The listing builds one solid part. Answer for the finished solid, in the listing's coordinates (mm). A direction names the side the tool comes from. Give positions to 0.01 mm unless a question says otherwise; leave off trailing zeros. Order: outer loops, then holes, each group sorted by start corner. A loop starts at its lowest first (then second) coordinate and runs counter-clockwise, first axis right, second up.
```python
from build123d import *

# Parameters (mm, degrees)
M5X0_8_1_AT_2_COUNT = 2
M5X0_8_1_AT_2_PITCH = 90.280227073


with BuildPart() as part:
    # 草图2 → 旋转4 (revolve)
    with BuildSketch(Plane(origin=(0, 0, 0), x_dir=(0, 0, -1), z_dir=(1, 0, 0)), mode=Mode.PRIVATE) as revolve_4_sk:
        Polygon((27.5, 94), (26, 94), (26, 96), (-26, 96), (-26, 94), (-27.5, 94), (-27.5, 90), (27.5, 90), align=None)
    revolve(revolve_4_sk.sketch.rotate(Axis((0, 90, -27.5), (0, 0, 1)), 90), axis=Axis((0, 90, -27.5), (0, 0, 1)))

    # 草图5 → M5x0.8 螺纹孔的螺纹孔钻头1 (revolve, cut)
    with BuildSketch(Plane(origin=(0, 90, 27.5), x_dir=(0, -1, 0), z_dir=(1, 0, 0))):
        Polygon((0, 0), (0, 16.2618073), (2.1, 15), (2.1, 0), align=None)
    m5x0_8_1 = revolve(axis=Axis((0, 90, 33.85), (0, 0, -1)), mode=Mode.SUBTRACT)

    # M5x0.8 螺纹孔的螺纹孔钻头1 at 2: M5x0.8 螺纹孔的螺纹孔钻头1 ×2
    with Locations(*[Vector(-0.6431998246516509, -0.765698364611082, 0) * (i * M5X0_8_1_AT_2_PITCH) for i in range(1, M5X0_8_1_AT_2_COUNT)]):
        add(m5x0_8_1, mode=Mode.SUBTRACT)

    # 镜向1: M5x0.8 螺纹孔的螺纹孔钻头1 across plane
    add(m5x0_8_1.mirror(Plane.XY), mode=Mode.SUBTRACT)

    # 镜向1 copy 1 sketch → 镜向1 copy 1 (revolve, cut)
    with BuildSketch(Plane(origin=(-58.068226223, 20.872577773, -27.5), x_dir=(0, -1, 0), z_dir=(1, 0, 0))):
        Polygon((0, 0), (0, -16.2618073), (2.1, -15), (2.1, 0), align=None)
    revolve(axis=Axis((-58.068226223, 20.872577773, -33.85), (0, 0, -1)), mode=Mode.SUBTRACT)


solid = part.part
```
1) Given P1, Ø5.5, axis at x = 0, y = 90, coming from the -Z side; P2, Ø1, axis at x = 1.5, z = 6.5, coming from the +Y side; P3, Ø2, axis at y = 93.5, z = 9, coming from the -X side; P4, Ø3, axis at x = 2, z = -18, coming from the -Y side, each flat-ended and moving along its own axis, determine where each tip first touches the part or whether it passes through.
Geometry says:
P1: stops at z = -27.5
P2: stops at y = 95.92
P3: stops at x = -5.45
P4: stops at y = 84.02
2) Find section B-B (x = -3.25). Write down the section's boundary in (y, z), then the cut area to 3 significant figures.
Geometry says:
outline: (84.96, -26) - (87.67, -26) - (87.67, -27.5) - (92.33, -27.5) - (92.33, -26) - (95.04, -26) - (95.04, 26) - (92.33, 26) - (92.33, 27.5) - (87.67, 27.5) - (87.67, 26) - (84.96, 26) - close
area: 539 mm2
3) A tool of negligible diameter and unlimited length cuts with its end or side. For faces 4 (the cylindrical face through (-0.09, 92.1, 20.1)), 5 (the cylindrical face through (0.867, 93.905, -26.74)), 6 (the flat face through (2, 92, -27.5)), from which of +Z, -Z, +X, -X, +Y, -Y can it reach the whole face along a straight path? Write none if from no direction.
Geometry says:
face 4: +Z
face 5: -Z
face 6: -Z, +X, -X, +Y, -Y
4) Straight lines are drawn through the part: probe 1 along X at (y, z) = (90, 18.25); probe 2 along Y at (x, z) = (0, -22); probe 3 along Z at (x, y) = (-3.5, 93). For each, find the intervals that lie inside material, in ascending order.
Geometry says:
probe 1: x = -6 to -2.1, 2.1 to 6
probe 2: y = 84 to 87.9, 92.1 to 96
probe 3: z = -26 to 26
5) Find section A-A (z = 13). Write down the section's boundary in (x, y).
Geometry says:
outline: circle Ø12 at (0, 90); hole circle Ø4.2 at (0, 90)
6) Find section D-D (y = 95.25). Write down the section's boundary in (x, z), then the cut area to 3 significant figures.
Geometry says:
outline: (-2.9, -26) - (2.9, -26) - (2.9, 26) - (-2.9, 26) - close
area: 302 mm2
7) For a pull along Y with two mould halves and no side action, classify faces 1 (the conical face through (-0.016, 90.364, 11.457)), 2 (the flat face through (-2, 92, 27.5)), 3 (the cylindrical face through (0.867, 93.905, 26.76)) as +Y half, -Y half, draft (parallel to the pull), parting line (faces both ways), or undercut.
Geometry says:
face 1: undercut
face 2: draft
face 3: parting line
8) Find section C-C (z = -9). Write down the section's boundary in (x, y), then the cut area to 3 significant figures.
Geometry says:
outline: circle Ø12 at (0, 90)
area: 113 mm2
